from build123d import *

# Parameters (mm, degrees)
F0_W     = 152.4
F0_H     = 101.6
F0_W_2   = 25.4
F0_H_2   = 81.28
F0_R     = 6.8811471087
F1_DEPTH = 19.05
F2_DEPTH = 3.81
F3_W     = 51.308
F3_H     = 88.9
F3_W_2   = 43.688
F3_H_2   = 81.28
F4_DEPTH = 3.81


with BuildPart() as f1:
    # F0 (on Top) → F1 (new body)
    with BuildSketch(Plane.XY):
        with Locations((-13.9326911301, 0.1037381589)):
            Rectangle(F0_W, F0_H)
        Polygon((-79.9726911301, -4.4682618411), (-79.9726911301, 40.7437381589), (-36.2846911301, 40.7437381589), (-26.1246911301, 40.7437381589), (-4.7886911301, 40.7437381589), (16.5473088699, 40.7437381589), (16.5473088699, 19.4077381589), (16.5473088699, -40.5362618411), (-26.1246911301, -40.5362618411), (-36.2846911301, -40.5362618411), (-79.9726911301, -40.5362618411), align=None, mode=Mode.SUBTRACT)
        with Locations((39.4073088699, 0.1037381589)):
            Rectangle(F0_W_2, F0_H_2, mode=Mode.SUBTRACT)
        with BuildLine():
            ThreePointArc((16.5473088699, 19.4077381589), (-4.7886911301, -1.9282618411), (-26.1246911301, 19.4077381589))
            Line((-26.1246911301, 19.4077381589), (-26.1246911301, -40.5362618411))
            Line((-26.1246911301, -40.5362618411), (16.5473088699, -40.5362618411))
            Line((16.5473088699, -40.5362618411), (16.5473088699, 19.4077381589))
        make_face()
        with Locations((-5.0076562911, -23.2165120542)):
            Circle(F0_R, mode=Mode.SUBTRACT)
        with BuildLine():
            Line((16.5473088699, 40.7437381589), (-4.7886911301, 40.7437381589))
            ThreePointArc((-4.7886911301, 40.7437381589), (10.2981391533, 34.4945684423), (16.5473088699, 19.4077381589))
            Line((16.5473088699, 19.4077381589), (16.5473088699, 40.7437381589))
        make_face()
        with BuildLine():
            Line((-4.7886911301, 40.7437381589), (-26.1246911301, 40.7437381589))
            Line((-26.1246911301, 40.7437381589), (-26.1246911301, 19.4077381589))
            ThreePointArc((-26.1246911301, 19.4077381589), (-19.8755214135, 34.4945684423), (-4.7886911301, 40.7437381589))
        make_face()
        Polygon((-26.1246911301, 40.7437381589), (-36.2846911301, 40.7437381589), (-36.2846911301, -40.5362618411), (-26.1246911301, -40.5362618411), (-26.1246911301, 19.4077381589), align=None)
    extrude(amount=F1_DEPTH)

    # F0 (on Top) → F2 (join)
    with BuildSketch(Plane.XY):
        Polygon((-36.2846911301, 40.7437381589), (-79.9726911301, 40.7437381589), (-79.9726911301, -4.4682618411), (-79.9726911301, -40.5362618411), (-36.2846911301, -40.5362618411), align=None)
        with BuildLine():
            ThreePointArc((16.5473088699, 19.4077381589), (10.2981391533, 34.4945684423), (-4.7886911301, 40.7437381589))
            ThreePointArc((-4.7886911301, 40.7437381589), (-19.8755214135, 34.4945684423), (-26.1246911301, 19.4077381589))
            ThreePointArc((-26.1246911301, 19.4077381589), (-4.7886911301, -1.9282618411), (16.5473088699, 19.4077381589))
        make_face()
        with Locations((-5.0076562911, -23.2165120542)):
            Circle(F0_R)
        with Locations((39.4073088699, 0.1037381589)):
            Rectangle(F0_W_2, F0_H_2)
    extrude(amount=F2_DEPTH)

    # F3 (on face) → F4 (cut)
    with BuildSketch(Plane.XY.offset(19.05)):
        with Locations((-58.1286911301, 0.1037381589)):
            Rectangle(F3_W, F3_H)
        with Locations((-58.1286911301, 0.1037381589)):
            Rectangle(F3_W_2, F3_H_2, mode=Mode.SUBTRACT)
        with Locations((-58.1286911301, 0.1037381589)):
            Rectangle(F3_W_2, F3_H_2)
    extrude(amount=-F4_DEPTH, mode=Mode.SUBTRACT)


solid = f1.part
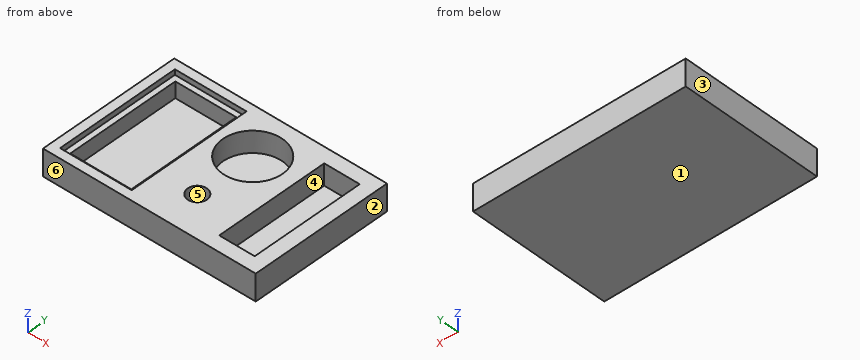
Model file for the job. Use its own axes, mm. Face numbers are marked on the shaded views. A direction names the side the tool comes from. Coordinates: 2 decimals unless noted, no trailing zeros. Loops run counter-clockwise (first coordinate to the right, second up) from the corner with the lowest first, then second, coordinate; pieces in that order, holes last. Notation, with made-up numbers: (35, 72.25) -> (43, 72.25) arc R17 cw to (43, 97.25) -> close; hole circle Ø9 at (34, 1.5). An arc over 180 degrees is marked (long way). Use one line per item in the form item = value. Start each with the question number.
(1) Cut at A-A on x = -75.5. Give the cut face in (y, z), and give its area (3 significant figures).
(2) Probe probe 1 along X at (y, z) = (-40.5, 6.75); probe 2 along X at (y, z) = (19, 9.5); probe 3 along Y at (x, z) = (45.5, 16.25). List the from-to ranges inside material, lowest first. Write a range as from..to.
(3) Pull direction X, two halves, no side cores. Call the marked faces 1, 2, 3 and 4: pulls with the +X half, pulls with the -X half, needs draft (parallel to the pull), parting line crosses it, or undercut.
(4) Cut at C-C on y = -25. Give the cut face in (x, z), and give its area (3 significant figures).
(5) Cut at D-D on x = 40.5. Give the cut face in (y, z), and give its area (3 significant figures).
(6) Tool access for the marked faces 5 and 6: list every direction of +Z, -Z, +X, -X, +Y, -Y with a clear straight run to the whole face (end or side of a thin tool).
(7) Cut at B-B on z = 13.25. Give the cut face in (x, y), and give its area (3 significant figures).
(8) Flat gauge pin, fed straight in: pin 1 (12.5 mm diameter, centred on x = -5.01, y = -23.22, fed in from +Z). Where does the tip first touch, or does it go through?
Values:
q1.outline = (-50.7, 0) -> (50.9, 0) -> (50.9, 19.05) -> (44.55, 19.05) -> (44.55, 15.24) -> (40.74, 15.24) -> (40.74, 3.81) -> (-40.54, 3.81) -> (-40.54, 15.24) -> (-44.35, 15.24) -> (-44.35, 19.05) -> (-50.7, 19.05) -> close
q1.area = 668 mm2
q2.probe_1 = -90.13..-79.97, -36.28..26.71, 52.11..62.27
q2.probe_2 = -90.13..-79.97, -36.28..-26.12, 16.54..26.71, 52.11..62.27
q2.probe_3 = -50.7..-40.54, 40.74..50.9
q3.face_1 = needs draft
q3.face_2 = pulls with the +X half
q3.face_3 = pulls with the -X half
q3.face_4 = undercut
q4.outline = (-90.13, 0) -> (62.27, 0) -> (62.27, 19.05) -> (52.11, 19.05) -> (52.11, 3.81) -> (26.71, 3.81) -> (26.71, 19.05) -> (1.64, 19.05) -> (1.64, 3.81) -> (-11.65, 3.81) -> (-11.65, 19.05) -> (-32.47, 19.05) -> (-32.47, 15.24) -> (-36.28, 15.24) -> (-36.28, 3.81) -> (-79.97, 3.81) -> (-79.97, 15.24) -> (-83.78, 15.24) -> (-83.78, 19.05) -> (-90.13, 19.05) -> close
q4.area = 1,620 mm2
q5.outline = (-50.7, 0) -> (50.9, 0) -> (50.9, 19.05) -> (40.74, 19.05) -> (40.74, 3.81) -> (-40.54, 3.81) -> (-40.54, 19.05) -> (-50.7, 19.05) -> close
q5.area = 697 mm2
q6.face_5 = +Z
q6.face_6 = +Z, -Z, +X, -X, -Y
q7.outline = (-90.13, -50.7) -> (62.27, -50.7) -> (62.27, 50.9) -> (-90.13, 50.9) -> close; hole (-79.97, -40.54) -> (-36.28, -40.54) -> (-36.28, 40.74) -> (-79.97, 40.74) -> close; hole circle Ø42.67 at (-4.79, 19.41); hole circle Ø13.76 at (-5.01, -23.22); hole (26.71, -40.54) -> (52.11, -40.54) -> (52.11, 40.74) -> (26.71, 40.74) -> close
q7.area = 8,290 mm2
q8.pin_1 = 3.81
